The listing builds one solid part. Answer for the finished solid, in the listing's coordinates (mm). Coordinates: 2 decimals unless noted, no trailing zeros. Loops run counter-clockwise (first coordinate to the right, second up) from the corner with the lowest first, then second, coordinate; pieces in that order, holes last. Notation, with made-up numbers: (18.5, 84.5) -> (47.5, 84.5) arc R19 cw to (47.5, 116.5) -> close; hole circle Ø1 at (-21.5, 72.25). An arc over 180 degrees is marked (long way). Answer in a Markdown table with one row per item.
```python
from build123d import *

# Parameters (mm, degrees)
SKETCH_1_W                  = 10
SKETCH_1_H                  = 20
SKETCH_1_W_2                = 7
SKETCH_1_H_2                = 17
EXTRUDE_1_DEPTH             = 250
HOLE_WIZARD_M61_D           = 6.6
HOLE_WIZARD_M61_CBORE_D     = 11
HOLE_WIZARD_M61_CBORE_DEPTH = 6.4
HOLE_WIZARD_1_D             = 10
HOLE_WIZARD_1_DEPTH         = 100


with BuildPart() as part:
    # Эскиз1 → Вытянуть-Тонкостенный1 (new body)
    with BuildSketch(Plane.XY):
        with Locations((5, 10)):
            Rectangle(SKETCH_1_W, SKETCH_1_H)
        with Locations((5, 10)):
            Rectangle(SKETCH_1_W_2, SKETCH_1_H_2, mode=Mode.SUBTRACT)
    extrude(amount=EXTRUDE_1_DEPTH)

    # Цековка для  винта с внутренним шестигранником M61 (through all)
    with Locations(Plane(origin=(10, 0, 0), x_dir=(0, 0, -1), z_dir=(1, 0, 0))):
        with Locations((-235, 10), (-125, 10), (-15, 10)):
            CounterBoreHole(HOLE_WIZARD_M61_D / 2, HOLE_WIZARD_M61_CBORE_D / 2, HOLE_WIZARD_M61_CBORE_DEPTH)

    # Отверстие1
    with Locations(Plane.ZY):
        with Locations((50, 10), (100, 10), (150, 10), (200, 10)):
            Hole(HOLE_WIZARD_1_D / 2, depth=HOLE_WIZARD_1_DEPTH)


solid = part.part
```
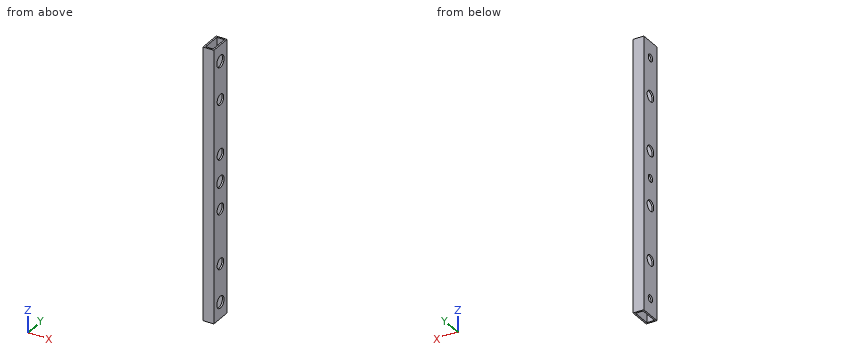
Item 1: A cutting plane is placed at B-B, the plane z = 50. Determine the outline of the cut face in (x, y).
Findings below:
| item | result |
|---|---|
| outline | (0, 0) -> (10, 0) -> (10, 5) -> (8.5, 5) -> (8.5, 1.5) -> (1.5, 1.5) -> (1.5, 5) -> (0, 5) -> close; (0, 15) -> (1.5, 15) -> (1.5, 18.5) -> (8.5, 18.5) -> (8.5, 15) -> (10, 15) -> (10, 20) -> (0, 20) -> close |
Item 2: A cutting plane is placed at C-C, the plane y = 10. Count the separate pieces of the cut face and the enclosed holes in it, plus the area to 3 significant figures.
Findings below:
| item | result |
|---|---|
| separate pieces | 16 |
| enclosed holes | 0 |
| area | 551 mm2 |
Item 3: A cutting plane is placed at D-D, the plane z = 235. Determine the outline of the cut face in (x, y).
Findings below:
| item | result |
|---|---|
| outline | (0, 0) -> (10, 0) -> (10, 4.5) -> (8.5, 4.5) -> (8.5, 1.5) -> (1.5, 1.5) -> (1.5, 6.7) -> (0, 6.7) -> close; (0, 13.3) -> (1.5, 13.3) -> (1.5, 18.5) -> (8.5, 18.5) -> (8.5, 15.5) -> (10, 15.5) -> (10, 20) -> (0, 20) -> close |
Item 4: Find the intervals of material crossed by probe 1 along Y at (x, z) = (9.2, 150); probe 2 along X at (y, z) = (9.25, 70.5); probe 3 along Y at (x, z) = (4.75, 169.5), in increasing order.
Findings below:
| item | result |
|---|---|
| probe 1 | y = 0 to 5, 15 to 20 |
| probe 2 | x = 0 to 1.5, 8.5 to 10 |
| probe 3 | y = 0 to 1.5, 18.5 to 20 |
Item 5: Flat-ended cylindrical pins translate along their axes: pin 1 Ø9 at (y, z) = (10, 15) entering from -X; pin 2 Ø10 at (y, z) = (10, 235) entering from +X; pin 3 Ø6 at (y, z) = (10, 15) entering from -X. Find the tip coordinate at first contact, or state that the pin passes through.
Findings below:
| item | result |
|---|---|
| pin 1 | stops at x = 0 |
| pin 2 | stops at x = 1.5 |
| pin 3 | passes through |
Item 6: A cutting plane is placed at A-A, the plane x = 5. Determine the outline of the cut face in (y, z).
Findings below:
| item | result |
|---|---|
| outline | (0, 0) -> (1.5, 0) -> (1.5, 250) -> (0, 250) -> close; (18.5, 0) -> (20, 0) -> (20, 250) -> (18.5, 250) -> close |
